from build123d import *

# Parameters (mm, degrees)
BOSS_EXTRUDE3_DEPTH            = 6.35
F_5_16_0_3125_DIAMETER_HOLE2_D = 7.9375
FILLET2_R                      = 19.05


with BuildPart() as part:
    # Sketch1 → Boss-Extrude3 (new body)
    with BuildSketch(Plane(origin=(0, 0, 0), x_dir=(1, 0, 0), z_dir=(0, 1, 0))):
        with BuildLine():
            Line((160.560790495, -59.070061434), (188.794553327, -136.64168728))
            Line((188.794553327, -136.64168728), (224.596842179, -123.610719819))
            Line((224.596842179, -123.610719819), (196.363079347, -46.039093974))
            Line((196.363079347, -46.039093974), (147.316678264, 88.71478551))
            ThreePointArc((147.316678264, 88.71478551), (95.182229706, 59.114314079), (85.197916699, 0))
            ThreePointArc((85.197916699, 0), (131.323386462, -18.761949266), (160.560790495, -59.070061434))
        make_face()
        with BuildLine():
            ThreePointArc((105.56875, 19.05), (114.038085826, 45.911301485), (136.382769163, 63.056980047))
            ThreePointArc((136.382769163, 63.056980047), (138.754781808, 68.14377758), (133.667984275, 70.515790225))
            ThreePointArc((133.667984275, 70.515790225), (107.536066474, 50.464064448), (97.63125, 19.05))
            ThreePointArc((97.63125, 19.05), (101.6, 15.08125), (105.56875, 19.05))
        make_face(mode=Mode.SUBTRACT)
    extrude(amount=BOSS_EXTRUDE3_DEPTH)

    # 5/16 (0.3125) Diameter Hole2 (through all)
    with Locations(Plane(origin=(0, 6.35, 0), x_dir=(1, 0, 0), z_dir=(0, 1, 0))):
        with Locations((152.4, 19.05), (182.805590742, -64.488673988), (200.180214023, -112.225059124)):
            Hole(F_5_16_0_3125_DIAMETER_HOLE2_D / 2)

    # Fillet2
    fillet2_edges = [part.edges().sort_by_distance(p)[0] for p in [
        (147.316678264, 3.175, -88.71478551),
        (224.596842179, 3.175, 123.610719819),
        (188.794553327, 3.175, 136.64168728),
        (85.197916699, 3.175, 0),
    ]]
    fillet(fillet2_edges, radius=FILLET2_R - 0.0001)  # a hair under: the kernel refuses the full size


solid = part.part
Input: part model. Units: mm. Frame: model coordinates. A direction names the side the tool comes from. Give positions to 0.01 mm unless a question says otherwise; leave off trailing zeros. Order: outer loops, then holes, each group sorted by start corner. A loop starts at its lowest first (then second) coordinate and runs counter-clockwise, first axis right, second up. Notation, with made-up numbers: M 49,13.5 L 86,13.5 A25 cw 86,44.5 Z; hole C 52,-8 d7. An arc over 180 degrees is marked long. Answer as a JSON object with one key per item and string values.
1. Reachability of faces 5 (the cylindrical face through (101.513, 3.131, -15.082)), 6 (the flat face through (171.27, 3.13, 88.49)) from +Z, -Z, +X, -X, +Y, -Y: full face, straight path, thin tool, end or side. Return the list, or none.
Result sheet:
{"face 5": "+Y, -Y", "face 6": "+Z, -X, +Y, -Y"}
2. First-contact query: P1, Ø2, axis at x = 145, y = 2, coming from the +Z side; P2, Ø2, axis at y = 2, z = 69, coming from the +X side; P3, Ø1, axis at y = 5.5, z = 15.5, coming from the -X side. Flat tips, straight axial feed; report the tip coordinate or a pass-through.
Result sheet:
{"P1": "z = 33.25", "P2": "x = 205.08", "P3": "x = 126.16"}
3. Pull-direction query (Z, two-part tool) for faces 1 (the cylindrical face through (135.496, 3.131, 22.239)), 2 (the cylindrical face through (142.886, 3.219, -84.139)), 3 (the cylindrical face through (217.356, 3.219, 120.465)), 4 (the cylindrical face through (183.666, 3.131, 68.363)); classes: +Z half, -Z half, draft (parallel to the pull), parting line (faces both ways), or undercut.
Result sheet:
{"face 1": "+Z half", "face 2": "-Z half", "face 3": "parting line", "face 4": "undercut"}
4. Cut plane D-D, the plane z = 14. Output: boundary loops of the cut face in (x, y), and give its area (3 significant figures).
Result sheet:
{"outline": "M 124.65,0 L 184.7,0 L 184.7,6.35 L 124.65,6.35 Z", "area": "381 mm²"}
5. Ray query, line 1 (X direction, y = 4.5, z = -35.5); line 2 (Z direction, x = 131, y = 4); line 3 (Z direction, x = 128, y = 3.25). Return the intervals inside material, ascending. Write a range as [from, to].
Result sheet:
{"line 1": "[84.51, 100.16], [108.55, 166.69]", "line 2": "[-85.41, -69.46], [-60.71, 18.51]", "line 3": "[-84.5, -68.08], [-59.02, 16.28]"}
6. Cut plane C-C, the plane y = 1. State how many separate pieces and enclosed holes the cut face has, and give its area (3 significant figures).
Result sheet:
{"separate pieces": "1", "enclosed holes": "4", "area": "11,200 mm²"}
7. Cut plane A-A, the plane z = -43. Output: boundary loops of the cut face in (x, y), and give its area (3 significant figures).
Result sheet:
{"outline": "M 86.78,0 L 103.15,0 L 103.15,6.35 L 86.78,6.35 Z; M 112.16,0 L 163.96,0 L 163.96,6.35 L 112.16,6.35 Z", "area": "433 mm²"}
8. Cut plane B-B, the plane x = 126. Output: boundary loops of the cut face in (y, z), and give its area (3 significant figures).
Result sheet:
{"outline": "M 0,-83.72 L 6.35,-83.72 L 6.35,-67.04 L 0,-67.04 Z; M 0,-57.73 L 6.35,-57.73 L 6.35,14.89 L 0,14.89 Z", "area": "567 mm²"}
